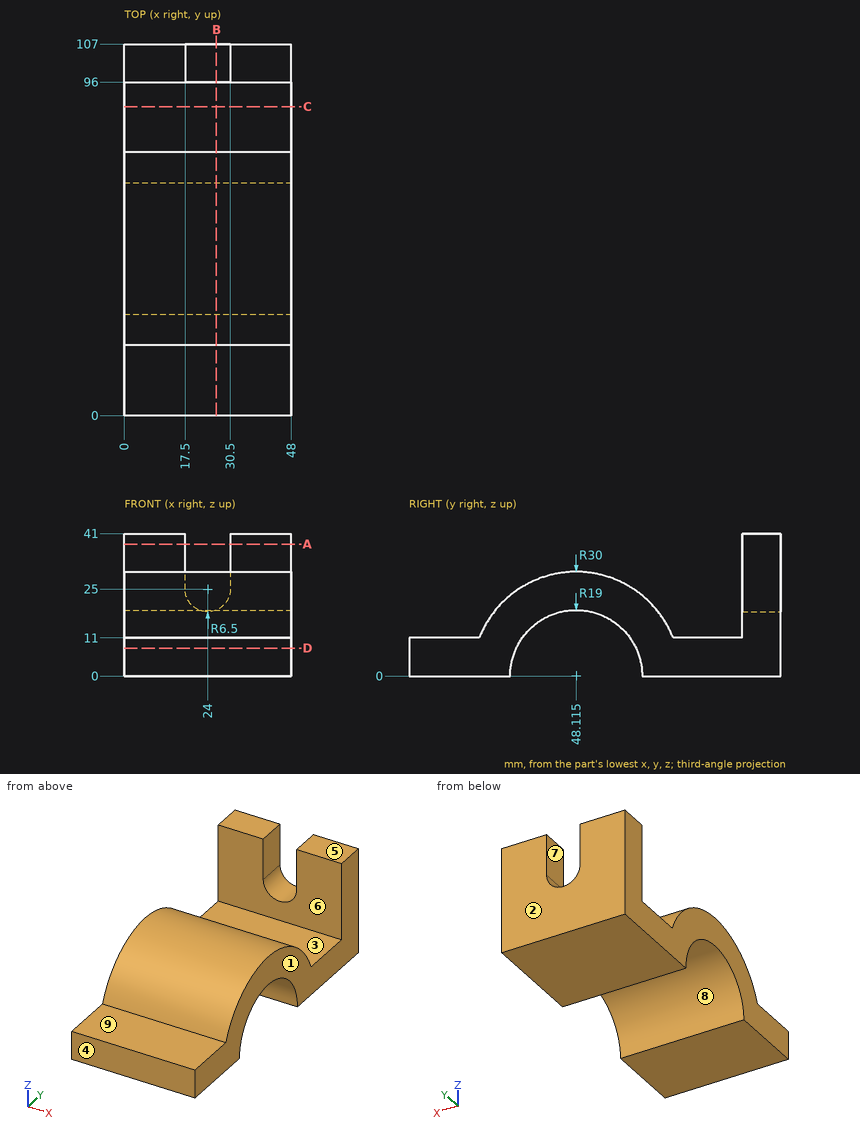
Source: three-view drawing plus pictorial views. Frame: mm from the lowest corner of the part. A direction names the side the tool comes from. Coordinates: 2 decimals unless noted, no trailing zeros. Write each loop counter-clockwise with the first axis right and the second up, starting at its lowest first coordinate (ties: lowest second). Pieces come first, ordered by that corner, then holes. Notation, with made-up numbers: (-17, 58.5) -> (12, 58.5) arc R22 cw to (12, 64.5) -> close; hole circle Ø8 at (-18.5, 33). An arc over 180 degrees is marked (long way). Answer as a JSON object with one key per item and string values.
1. First-contact query: P1, Ø3, axis at x = 6, y = 81.5, coming from the +Z side; P2, Ø8, axis at x = 41.5, z = 27, coming from the -Y side (1 decimal); P3, Ø9, axis at x = 25, z = 24.5, coming from the -Y side (1 decimal). Flat tips, straight axial feed; report the tip coordinate or a pass-through.
Result set:
{"P1": "stops at z = 11", "P2": "stops at y = 28.9", "P3": "stops at y = 25.8"}
2. Section B-B on x = 26.5. Return the cut outline in (y, z) (1 decimal), then the cut area to 3 significant figures.
Result set:
{"outline": "(0, 0) -> (29.1, 0) arc R19 cw to (67.1, 0) -> (107, 0) -> (107, 19) -> (96, 19) -> (96, 11) -> (76, 11) arc R30 ccw to (20.2, 11) -> (0, 11) -> close", "area": "1,470 mm2"}
3. Mould query, pull axis Y, two halves, no side actions, for the marked faces 1, 2, 3 and 4. Classes: released by +Y, released by -Y, zero draft, split by the parting line, or undercut.
Result set:
{"face 1": "zero draft", "face 2": "released by +Y", "face 3": "undercut", "face 4": "released by -Y"}
4. Section D-D on z = 8. Return the cut outline in (x, y).
Result set:
{"outline": "(0, 0) -> (48, 0) -> (48, 30.88) -> (0, 30.88) -> close; (0, 65.35) -> (48, 65.35) -> (48, 107) -> (0, 107) -> close"}
5. Material intervals for line 1 (Y direction, x = 19, z = 13); line 2 (X direction, y = 98.5, z = 25); line 3 (Y direction, x = 41, z = 3), sorted ascending. Write a range as from..to.
Result set:
{"line 1": "y = 21.08..34.26, 61.97..75.15, 96..107", "line 2": "x = 0..17.5, 30.5..48", "line 3": "y = 0..29.35, 66.88..107"}
6. Access query for the marked faces 5, 6, 7, 8 and 9. Directions: +Z, -Z, +X, -X, +Y, -Y. A direction counts if a zero-diameter tool reaches every point of the face in a straight line with its end or side. Return the directions, or none.
Result set:
{"face 5": "+Z, +X, -X, +Y, -Y", "face 6": "+Z, +X, -X", "face 7": "+Z, +Y", "face 8": "-Z, +X, -X", "face 9": "+Z, +X, -X, -Y"}
7. Section C-C on y = 89. Return the cut outline in (x, z).
Result set:
{"outline": "(0, 0) -> (48, 0) -> (48, 11) -> (0, 11) -> close"}
8. Section A-A on z = 38. Return the cut outline in (x, y), then the cut area to 3 significant figures.
Result set:
{"outline": "(0, 96) -> (17.5, 96) -> (17.5, 107) -> (0, 107) -> close; (30.5, 96) -> (48, 96) -> (48, 107) -> (30.5, 107) -> close", "area": "385 mm2"}
